Here's how the part is built. I have some questions about the finished solid (model axes, mm). A direction names the side the tool comes from. Give positions to 0.01 mm unless a question says otherwise; leave off trailing zeros. Write each loop counter-clockwise with the first axis right and the second up, starting at its lowest first coordinate (ties: lowest second). Pieces come first, ordered by that corner, then holes. Notation, with made-up numbers: (3.25, 39.25) -> (15.25, 39.25) arc R22 ccw to (15.25, 68.25) -> close; hole circle Ø3 at (-12, 35.5). An arc over 180 degrees is marked (long way). Answer as CSV lines item,"result". Start each with the question number.
from build123d import *

# Parameters (mm, degrees)
SKETCH_1_R          = 25
SKETCH_1_W          = 81
SKETCH_1_H          = 42
SKETCH_1_R_2        = 2.5
EXTRUDE_1_DEPTH     = 5
SKETCH_3_W          = 8.1
SKETCH_3_H          = 6.6
SKETCH_3_R          = 1.575
CUT_EXTRUDE_1_DEPTH = 2
SKETCH_3_2_R        = 1.575
CUT_EXTRUDE_2_DEPTH = 49.280430818
SKETCH_4_W          = 8
SKETCH_4_H          = 2.9
EXTRUDE_2_DEPTH     = 42
SKETCH_1_3_R        = 2.5
CUT_EXTRUDE_3_DEPTH = 42
EXTRUDE_START       = 21
SKETCH_5_W          = 11
SKETCH_5_H          = 2.9
EXTRUDE_3_DEPTH     = 5
SKETCH_5_W_2        = 12
EXTRUDE_3_2_DEPTH   = 5
CUT_EXTRUDE_4_REACH = 87.138
CHAMFER_1_SIZE      = 2
EXTRUDE_4_DEPTH     = 15
EXTRUDE_4_2_DEPTH   = 15
EXTRUDE_START_2     = -15
EXTRUDE_5_DEPTH     = 7.9
EXTRUDE_6_DEPTH     = 15
EXTRUDE_7_DEPTH     = 7.9
FILLET_1_R          = 5


# Read off the part's stored shape, not the designer's step: the extrude step
with BuildPart() as part:
    # Sketch 1 → Extrude 1 (new body)
    # profile 1 of 2: a face of its own
    with BuildSketch(Plane(origin=(0, 0, 0), x_dir=(1, 0, 0), z_dir=(0, 1, 0))):
        Circle(SKETCH_1_R)
    # profile 2 of 2: a face of its own
    with BuildSketch(Plane(origin=(0, 0, 0), x_dir=(1, 0, 0), z_dir=(0, 1, 0))):
        with Locations((-0.5, 0)):
            Rectangle(SKETCH_1_W, SKETCH_1_H)
        with Locations(Location((35, 16, 0), (0, 0, 270))):
            Circle(SKETCH_1_R_2, mode=Mode.SUBTRACT)
        with Locations(Location((35, -16, 0), (0, 0, 270))):
            Circle(SKETCH_1_R_2, mode=Mode.SUBTRACT)
        with Locations(Location((-36, 14.75, 0), (0, 0, 270))):
            Circle(SKETCH_1_R_2, mode=Mode.SUBTRACT)
        with Locations(Location((-36, -14.75, 0), (0, 0, 270))):
            Circle(SKETCH_1_R_2, mode=Mode.SUBTRACT)
    extrude(amount=EXTRUDE_1_DEPTH)

    # Sketch 3 → Cut-Extrude 1 (cut)
    # profile 1 of 2: a face of its own
    with BuildSketch(Plane(origin=(0, 5, 0), x_dir=(1, 0, 0), z_dir=(0, 1, 0))):
        with Locations((-6.75, -14)):
            Rectangle(SKETCH_3_W, SKETCH_3_H)
        with Locations(Location((-6.75, -14, 0), (0, 0, 90))):
            Circle(SKETCH_3_R, mode=Mode.SUBTRACT)
    # profile 2 of 2: a face of its own
    with BuildSketch(Plane(origin=(0, 5, 0), x_dir=(1, 0, 0), z_dir=(0, 1, 0))):
        with Locations((-6.75, 14)):
            Rectangle(SKETCH_3_W, SKETCH_3_H)
        with Locations(Location((-6.75, 14, 0), (0, 0, 270))):
            Circle(SKETCH_3_R, mode=Mode.SUBTRACT)
    extrude(amount=-CUT_EXTRUDE_1_DEPTH, mode=Mode.SUBTRACT)

    # Sketch 3_2 → Cut-Extrude 2 (cut, through all)
    with BuildSketch(Plane(origin=(0, 5, 0), x_dir=(1, 0, 0), z_dir=(0, 1, 0))):
        with Locations(Location((-6.75, 14, 0), (0, 0, 270))):
            Circle(SKETCH_3_2_R)
        with Locations(Location((-6.75, -14, 0), (0, 0, 270))):
            Circle(SKETCH_3_2_R)
    extrude(amount=-CUT_EXTRUDE_2_DEPTH, mode=Mode.SUBTRACT)

    # Sketch 4 → Extrude 2 (add)
    with BuildSketch(Plane.XY.offset(21)):
        with Locations((36, 6.45)):
            Rectangle(SKETCH_4_W, SKETCH_4_H)
        with Locations((-37, 6.45)):
            Rectangle(SKETCH_4_W, SKETCH_4_H)
    extrude(amount=-EXTRUDE_2_DEPTH)

    # Sketch 1_3 → Cut-Extrude 3 (cut)
    with BuildSketch(Plane(origin=(0, 0, 0), x_dir=(1, 0, 0), z_dir=(0, 1, 0))):
        with Locations(Location((35, 16, 0), (0, 0, 270))):
            Circle(SKETCH_1_3_R)
        with Locations(Location((35, -16, 0), (0, 0, 270))):
            Circle(SKETCH_1_3_R)
        with Locations(Location((-36, 14.75, 0), (0, 0, 180))):
            Circle(SKETCH_1_3_R)
        with Locations(Location((-36, -14.75, 0), (0, 0, 180))):
            Circle(SKETCH_1_3_R)
    extrude(amount=CUT_EXTRUDE_3_DEPTH, mode=Mode.SUBTRACT)


with BuildPart() as body_2:
    # Sketch 5 → Extrude 3 (new body)
    with BuildSketch(Plane.XY.offset(EXTRUDE_START)):
        with Locations((26.5, 6.45)):
            Rectangle(SKETCH_5_W, SKETCH_5_H)
    extrude_3 = extrude(amount=-EXTRUDE_3_DEPTH)


with BuildPart() as body_3:
    # Sketch 5 → Extrude 3 2 (new body)
    with BuildSketch(Plane.XY.offset(EXTRUDE_START)):
        with Locations((-27, 6.45)):
            Rectangle(SKETCH_5_W_2, SKETCH_5_H)
    extrude_3_2 = extrude(amount=-EXTRUDE_3_2_DEPTH)



with BuildPart() as part_1:
    add(part.part)

    # Mirror 2: Extrude 3, Extrude 3 2 across plane
    add(extrude_3.mirror(Plane(origin=(0, 0, 0), x_dir=(1, 0, 0), z_dir=(0, 0, -1))))
    add(extrude_3_2.mirror(Plane(origin=(0, 0, 0), x_dir=(1, 0, 0), z_dir=(0, 0, -1))))

    # Cut-Extrude 4: up to this face of the body (flat: up to its plane)
    cut_extrude_4_end = Plane(part_1.part.faces().sort_by_distance((32, 6.45, 2.5))[0])
    # Sketch 6 → Cut-Extrude 4 (cut, up to the picked face)
    with BuildSketch(Plane.ZY.offset(41), mode=Mode.PRIVATE) as cut_extrude_4_sk1:
        with BuildLine():
            Line((11.041960784, 8.971428571), (-11.041960784, 8.971428571))
            ThreePointArc((-11.041960784, 8.971428571), (-8.690257734, 7.239234925), (-6.072727273, 5.943265655))
            ThreePointArc((-6.072727273, 5.943265655), (0, 4.8), (6.072727273, 5.943265655))
            ThreePointArc((6.072727273, 5.943265655), (8.690257734, 7.239234925), (11.041960784, 8.971428571))
        make_face()
    cut_extrude_4_tool1 = split(extrude(cut_extrude_4_sk1.sketch, amount=-CUT_EXTRUDE_4_REACH, mode=Mode.PRIVATE), bisect_by=cut_extrude_4_end, keep=Keep.BOTH, mode=Mode.PRIVATE)
    add(cut_extrude_4_tool1.solids().sort_by(Axis((-41, 7.283597, 0), (1, 0, 0)))[0], mode=Mode.SUBTRACT)

    # Chamfer 1
    chamfer_1_edges = [part_1.edges().sort_by_distance(p)[0] for p in [
        (-41, 3.95, 21),
        (-41, 3.95, -21),
        (40, 3.95, -21),
        (40, 3.95, 21),
    ]]
    chamfer(chamfer_1_edges, length=CHAMFER_1_SIZE)



with BuildPart() as body_4:
    # Sketch 9 → Extrude 4 (new body)
    with BuildSketch(Plane.XZ):
        with BuildLine():
            Line((33, 26), (23.72846392, 26))
            ThreePointArc((23.72846392, 26), (24.88485791, 24.895458357), (25.989891949, 23.739534884))
            ThreePointArc((25.989891949, 23.739534884), (27.687521221, 22.340851231), (29.708138181, 21.471732017))
            ThreePointArc((29.708138181, 21.471732017), (30.719571772, 21.268231436), (31.749015733, 21.2))
            Line((31.749015733, 21.2), (37.8, 21.2))
            Line((37.8, 21.2), (33, 26))
        make_face()
    extrude(amount=-EXTRUDE_4_DEPTH)


with BuildPart() as body_5:
    # Sketch 9 → Extrude 4 2 (new body)
    with BuildSketch(Plane.XZ):
        with BuildLine():
            Line((33, -26), (37.8, -21.2))
            Line((37.8, -21.2), (31.749015733, -21.2))
            ThreePointArc((31.749015733, -21.2), (30.719571772, -21.268231436), (29.708138181, -21.471732017))
            ThreePointArc((29.708138181, -21.471732017), (27.687521221, -22.340851231), (25.989891949, -23.739534884))
            ThreePointArc((25.989891949, -23.739534884), (24.88485791, -24.895458357), (23.72846392, -26))
            Line((23.72846392, -26), (33, -26))
        make_face()
    extrude(amount=-EXTRUDE_4_2_DEPTH)


with BuildPart() as part_2:
    add(part_1.part)

    add(body_4.part)  # Extrude 5 merges body 4
    # Sketch 10 → Extrude 5 (add)
    with BuildSketch(Plane(origin=(0, 15, 0), x_dir=(1, 0, 0), z_dir=(0, 1, 0)).offset(EXTRUDE_START_2)):
        with BuildLine():
            Line((21, -21), (23.72846392, -26))
            ThreePointArc((23.72846392, -26), (24.88485791, -24.895458357), (25.989891949, -23.739534884))
            ThreePointArc((25.989891949, -23.739534884), (28.601924052, -21.863066908), (31.749015733, -21.2))
            Line((31.749015733, -21.2), (37.8, -21.2))
            Line((37.8, -21.2), (38, -21))
            Line((38, -21), (32, -21))
            Line((32, -21), (21, -21))
        make_face()
    extrude_5 = extrude(amount=EXTRUDE_5_DEPTH)


with BuildPart() as body_3_1:
    add(body_3.part)

    add(part_2.part)  # Extrude 6 merges part
    # Sketch 11 → Extrude 6 (add)
    with BuildSketch(Plane.XZ.offset(EXTRUDE_START_2)):
        with BuildLine():
            Line((-41, 23), (-41, 20.45))
            Line((-41, 20.45), (-40.520827978, 20.45))
            ThreePointArc((-40.520827978, 20.45), (-40.024975712, 20.455165886), (-39.5293387, 20.4706613))
            Line((-39.5293387, 20.4706613), (-39, 21))
            Line((-39, 21), (-35.43383476, 21))
            ThreePointArc((-35.43383476, 21), (-31.171725667, 22.363148102), (-27.240108871, 24.5))
            Line((-27.240108871, 24.5), (-41, 24.5))
            Line((-41, 24.5), (-41, 23))
        make_face()
        with BuildLine():
            Line((-39, 21), (-39.5293387, 20.4706613))
            ThreePointArc((-39.5293387, 20.4706613), (-39.301113021, 20.481274846), (-39.072999743, 20.494078772))
            ThreePointArc((-39.072999743, 20.494078772), (-38.358018151, 20.54847571), (-37.644999743, 20.624386527))
            ThreePointArc((-37.644999743, 20.624386527), (-36.534990206, 20.786132091), (-35.43383476, 21))
            Line((-35.43383476, 21), (-39, 21))
        make_face()
    extrude_6 = extrude(amount=EXTRUDE_6_DEPTH)

    # Extrude 7 outline → Extrude 7 (add)
    with BuildSketch(Plane(origin=(0, 0, 0), x_dir=(1, 0, 0), z_dir=(0, 1, 0))):
        with BuildLine():
            Line((-39.5293387, -20.4706613), (-41, -19))
            Line((-41, -19), (-41, -20.45))
            Line((-41, -20.45), (-40.520827978, -20.45))
            ThreePointArc((-40.520827978, -20.45), (-40.024975712, -20.455165886), (-39.5293387, -20.4706613))
        make_face()
        with BuildLine():
            Line((-21, -21), (-35.43383476, -21))
            ThreePointArc((-35.43383476, -21), (-31.171725667, -22.363148102), (-27.240108871, -24.5))
            Line((-27.240108871, -24.5), (-21, -21))
        make_face()
    extrude_7 = extrude(amount=EXTRUDE_7_DEPTH)

    # Mirror 3: Extrude 5, Extrude 6, Extrude 7 across plane
    add(extrude_5.mirror(Plane(origin=(0, 0, 0), x_dir=(1, 0, 0), z_dir=(0, 0, -1))))
    add(extrude_6.mirror(Plane(origin=(0, 0, 0), x_dir=(1, 0, 0), z_dir=(0, 0, -1))))
    add(extrude_7.mirror(Plane(origin=(0, 0, 0), x_dir=(1, 0, 0), z_dir=(0, 0, -1))))


with BuildPart() as body_2_1:
    add(body_2.part)

    # Combine 1: union body 3, body 5
    add(body_3_1.part)
    add(body_5.part)

    # Fillet 1
    fillet_1_edges = [body_2_1.edges().sort_by_distance(p)[0] for p in [
        (32, 6.45, 16),
        (-33, 6.45, 16),
        (-33, 6.45, -16),
        (32, 6.45, -16),
    ]]
    fillet(fillet_1_edges, radius=FILLET_1_R)


solid = body_2_1.part
Item 1: If we section it at C-C (z = 8.5): Please give me the cut outline in (x, y).
Item 2: If I drill on line 1 (X direction, y = 4, z = -15); line 2 (Z direction, x = -30, y = 6.5); line 3 (Z direction, x = 35, y = 6), over which ranges is the centre line in solid material (lowest first)? Write a range as [from, to].
Item 3: If we section it at A-A (y = 11): Please give me the cut outline in (x, z) (3 decimals).
Item 4: I'm going to push flat-ended pins straight in: pin 1 (5.5 mm diameter, centred on x = -7.5, z = -15, fed in from +Y); pin 2 (3 mm diameter, centred on x = -6.75, z = 14, fed in from -Y); pin 3 (3 mm diameter, centred on x = -12.5, y = 2.5, fed in from -Z); pin 4 (1.5 mm diameter, centred on x = 18.5, y = 3.5, fed in from -Z). Where does each tip first touch, or does it pass through?
Item 5: If we section it at D-D (x = -18.5): Please give me the cut outline in (y, z), and give its area (3 significant figures).
Item 6: If we section it at B-B (x = -6.75): Please give me the cut outline in (y, z) (1 decimal).
Item 7: For faces 1 (the face through (30, 6, -15)), 2 (the face through (31, 15, -24)), 3 (the face through (-34, 8, -24.5)), 4 (the face through (35, 11, 21.2)), which set-ups out of +Z, -Z, +X, -X, +Y, -Y let a thin tool reach every point of the face, with its end or its side?
Item 8: We'd pull the mould along X, two halves only. Please class faces 5 (the face through (40, 4, 0)), 6 (the face through (-24.164, 3.895, 22.774)), 7 (the face through (28, 7, -26)): released by +X, released by -X, zero draft, split by the parting line, or undercut.
Final values:
1,outline,"(-41, 0) -> (40, 0) -> (40, 7.9) -> (32, 7.9) -> (32, 5) -> (-33, 5) -> (-33, 7.13) -> (-41, 7.13) -> close"
2,line 1,"[-41, -38.49], [-33.51, -10.8], [-2.7, 32.71], [37.29, 40]"
2,line 2,"[-24.5, -15.58], [15.58, 24.5]"
2,line 3,"[-24, -18.5], [-13.5, 13.5], [18.5, 24]"
3,outline,"(-41, -24.5) -> (-27.24, -24.5) arc R23.8 ccw to (-39.073, -20.494) arc R23.8 ccw to (-39.529, -20.471) arc R23.8 ccw to (-40.521, -20.45) -> (-41, -20.45) -> close; (-41, 20.45) -> (-40.521, 20.45) arc R23.8 ccw to (-39.529, 20.471) arc R23.8 ccw to (-39.073, 20.494) arc R23.8 ccw to (-27.24, 24.5) -> (-41, 24.5) -> close; (23.728, -26) -> (33, -26) -> (37.8, -21.2) -> (31.749, -21.2) arc R7.8 ccw to (25.99, -23.74) arc R35.2 cw to start; (23.728, 26) arc R35.2 cw to (25.99, 23.74) arc R7.8 ccw to (31.749, 21.2) -> (37.8, 21.2) -> (33, 26) -> close"
4,pin 1,"y = 5"
4,pin 2,"through"
4,pin 3,"z = -22.45"
4,pin 4,"z = -21"
5,outline,"(0, -21) -> (5, -21) -> (5, -2.58) arc R16.7 cw to (5, 2.58) -> (5, 21) -> (0, 21) -> close"
5,area,"209 mm2"
6,outline,"(0, -24.1) -> (5, -24.1) -> (5, -17.3) -> (3, -17.3) -> (3, -15.6) -> (0, -15.6) -> close; (0, -12.4) -> (3, -12.4) -> (3, -10.7) -> (5, -10.7) -> (5, -2.6) arc R16.7 cw to (5, 2.6) -> (5, 10.7) -> (3, 10.7) -> (3, 12.4) -> (0, 12.4) -> close; (0, 15.6) -> (3, 15.6) -> (3, 17.3) -> (5, 17.3) -> (5, 24.1) -> (0, 24.1) -> close"
7,face 1,"+Y"
7,face 2,"+Z, -Z, +X, -X, +Y"
7,face 3,"-Z, -X, +Y, -Y"
7,face 4,"+X, +Y"
8,face 5,"released by +X"
8,face 6,"undercut"
8,face 7,"zero draft"
